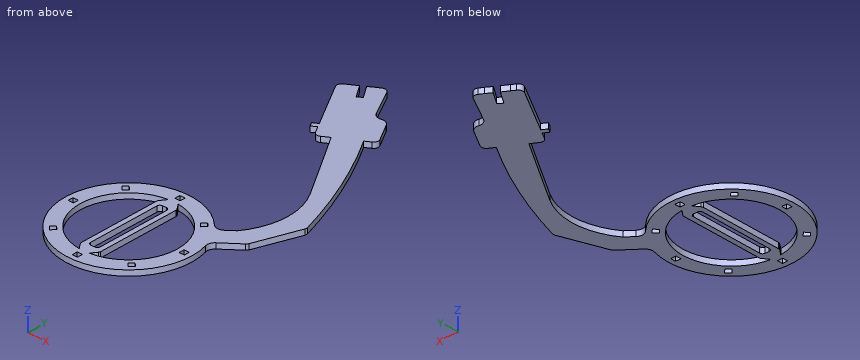
Autodesk Inventor part; units mm, degrees
ref_plane "YZ Plane" through (0, 0, 0) normal (1, 0, 0) x (0, 1, 0)
ref_plane "XZ Plane" through (0, 0, 0) normal (0, 1, 0) x (-1, 0, 0)
ref_plane "XY Plane" through (0, 0, 0) normal (0, 0, 1) x (1, 0, 0)
sketch "Sketch1" plane through (0, 0, 0) normal (0, 0, 1) x (1, 0, 0)
  circle A0 centre (0, 0) radius 65
  dimension "d0" = 130
extrude "Extrusion1" add sketch "Sketch1" along normal blind 5.5
sketch "Sketch5" plane through (0, 0, 5.5) normal (0, 0, 1) x (1, 0, 0)
  line L0 (54.5, 2.75) -> (60, 2.75)
  line L1 (60, 2.75) -> (60, -2.75)
  line L2 (60, -2.75) -> (54.5, -2.75)
  line L3 (54.5, -2.75) -> (54.5, 2.75)
  line L4 (36.5928, 40.4819) -> (40.4819, 44.371)
  line L5 (40.4819, 44.371) -> (44.371, 40.4819)
  line L6 (44.371, 40.4819) -> (40.4819, 36.5928)
  line L7 (40.4819, 36.5928) -> (36.5928, 40.4819)
  line L8 (-2.75, 54.5) -> (-2.75, 60)
  line L9 (-2.75, 60) -> (2.75, 60)
  line L10 (2.75, 60) -> (2.75, 54.5)
  line L11 (2.75, 54.5) -> (-2.75, 54.5)
  line L12 (-40.4819, 36.5928) -> (-44.371, 40.4819)
  line L13 (-44.371, 40.4819) -> (-40.4819, 44.371)
  line L14 (-40.4819, 44.371) -> (-36.5928, 40.4819)
  line L15 (-36.5928, 40.4819) -> (-40.4819, 36.5928)
  line L16 (-54.5, -2.75) -> (-60, -2.75)
  line L17 (-60, -2.75) -> (-60, 2.75)
  line L18 (-60, 2.75) -> (-54.5, 2.75)
  line L19 (-54.5, 2.75) -> (-54.5, -2.75)
  line L20 (-36.5928, -40.4819) -> (-40.4819, -44.371)
  line L21 (-40.4819, -44.371) -> (-44.371, -40.4819)
  line L22 (-44.371, -40.4819) -> (-40.4819, -36.5928)
  line L23 (-40.4819, -36.5928) -> (-36.5928, -40.4819)
  line L24 (2.75, -54.5) -> (2.75, -60)
  line L25 (2.75, -60) -> (-2.75, -60)
  line L26 (-2.75, -60) -> (-2.75, -54.5)
  line L27 (-2.75, -54.5) -> (2.75, -54.5)
  line L28 (40.4819, -36.5928) -> (44.371, -40.4819)
  line L29 (44.371, -40.4819) -> (40.4819, -44.371)
  line L30 (40.4819, -44.371) -> (36.5928, -40.4819)
  line L31 (36.5928, -40.4819) -> (40.4819, -36.5928)
  point P0 (0, 0)
  dimension "d30" = 5.5
  dimension "d31" = 5.5
  dimension "d34" = 360
extrude "Extrusion5" cut sketch "Sketch5" against normal blind 10
sketch "Sketch7" plane through (0, 0, 5.5) normal (0, 0, 1) x (1, 0, 0)
  circle A0 centre (0, 0) radius 65
  line L0 (51.1247, 40.1406) -> (64.8175, 50.8915)
  line L1 (60.6454, 23.3909) -> (84.0046, 41.7313)
  line L2 (84.0046, 41.7313) -> (101.175, 89.1614)
  arc A1 (68.2492, 128.5806) -> (22.61, 201.3724) centre (-8338.3582, -5091.5201) ccw
  arc A2 (101.175, 89.1614) -> (44.4638, 214.134) centre (-401.1925, -63.4539) ccw
  arc A3 (64.8175, 50.8915) -> (68.2492, 128.5806) centre (9.7334, 92.245) ccw
  line L3 (-9.0847, 275.4971) -> (0.0597, 261.7096)
  line L4 (0.0597, 261.7096) -> (-4.5238, 258.6697)
  line L5 (-4.5238, 258.6697) -> (-13.846, 272.7251)
  line L6 (-20.4878, 268.8466) -> (-13.846, 272.7251)
  line L7 (-9.0847, 275.4971) -> (-3.3614, 279.1755)
  line L8 (-20.4878, 268.8466) -> (-29.1232, 263.8039)
  line L9 (-3.3614, 279.1755) -> (5.4134, 283.9717)
  line L10 (11.2184, 194.7202) -> (22.61, 201.3724)
  line L11 (44.4638, 214.134) -> (54.3957, 219.9338)
  line L12 (4.4881, 206.2457) -> (-0.6932, 203.2201)
  line L13 (-0.6932, 203.2201) -> (-3.2145, 207.5378)
  line L14 (-3.2145, 207.5378) -> (1.9667, 210.5634)
  line L15 (-29.1232, 263.8039) -> (1.9667, 210.5634)
  line L16 (4.4881, 206.2457) -> (11.2184, 194.7202)
  line L17 (54.3957, 219.9338) -> (37.2403, 249.3118)
  line L18 (37.2403, 249.3118) -> (27.3211, 243.8901)
  line L19 (27.3211, 243.8901) -> (5.4134, 283.9717)
  dimension "d40" = 250
  dimension "d41" = 20
  dimension "d50" = 5.5
  dimension "d53" = 10
  dimension "d54" = 80
  dimension "d55" = 50
  dimension "d56" = 10
  dimension "d57" = 6
  dimension "d58" = 5
extrude "Extrusion6" add sketch "Sketch7" against normal blind 5.5 contours A0 L0 A3 A1 L10 L16 L12 L13 L14 L15 L8 L6 L5 L4 L3 L7 L9 L19 L18 L17 L11 A2 L2 L1
sketch "Sketch8" plane through (0, 0, 5.5) normal (0, 0, 1) x (1, 0, 0)
  circle A0 centre (0, 0) radius 50
  line L0 (10, 43) -> (10, -43)
  line L1 (-10, -43) -> (-10, 43)
  line L2 (5, 40) -> (-5, 40)
  line L3 (-5, 40) -> (-5, -40)
  line L4 (-5, -40) -> (5, -40)
  line L5 (5, -40) -> (5, 40)
  line L6 (10, -43) -> (5, -49.7494)
  line L7 (-10, -43) -> (-5, -49.7494)
  line L8 (-10, 43) -> (-5, 49.7494)
  line L9 (5, 49.7494) -> (10, 43)
  dimension "d44" = 100
  dimension "d45" = 10
  dimension "d46" = 80
extrude "Extrusion7" cut sketch "Sketch8" against normal blind 5.5 contours A0 L6 L0 L9 | L8 L1 L7 A0 | L5 L4 L3 L2
fillet "Fillet1" radius 3 8 edges at (10, 43, 2.75) (10, -43, 2.75) (-5, 40, 2.75) (-10, -43, 2.75) (5, 40, 2.75) (-10, 43, 2.75) (-5, -40, 2.75) (5, -40, 2.75)
fillet "Fillet2" radius 5 2 edges at (101.175, 89.1614, 2.75) (84.0046, 41.7313, 2.75)
fillet "Fillet3" radius 8 2 edges at (60.6454, 23.3909, 2.75) (51.1247, 40.1406, 2.75)
fillet "Fillet4" radius 5 4 edges at (54.3957, 219.9338, 2.75) (11.2184, 194.7202, 2.75) (5.4134, 283.9717, 2.75) (-29.1232, 263.8039, 2.75)
fillet "Fillet5" radius 8 2 edges at (27.3211, 243.8901, 2.75) (37.2403, 249.3118, 2.75)
properties part number "base"
Verification items for the finished model (mm, model axes). Coordinates: 2 decimals unless noted, no trailing zeros. Loops run counter-clockwise (first coordinate to the right, second up) from the corner with the lowest first, then second, coordinate; pieces in that order, holes last. Notation, with made-up numbers: (14.5, 30.5) -> (53.5, 30.5) arc R10 ccw to (53.5, 42.5) -> close; hole circle Ø3 at (21, 62.25). An arc over 180 degrees is marked (long way). Write each question's results on one line, items separated by ' | '.
Item 1: Section check A-A, the plane y = -20. Enter the section's corners in (x, z), plus the area to 3 significant figures.
Found:
outline: (-61.85, 0) -> (-45.83, 0) -> (-45.83, 5.5) -> (-61.85, 5.5) -> close; (-10, 0) -> (-5, 0) -> (-5, 5.5) -> (-10, 5.5) -> close; (5, 0) -> (10, 0) -> (10, 5.5) -> (5, 5.5) -> close; (45.83, 0) -> (61.85, 0) -> (61.85, 5.5) -> (45.83, 5.5) -> close | area: 231 mm2
Item 2: Material ranges on L1, parallel to X at y = 57, z = 3.5; L2, parallel to Y at x = 23.5, z = 1.25; L3, parallel to Y at x = -42.5, z = 4.05, recorded low to high.
Found:
L1: x = -31.24 to -2.75, 2.75 to 31.24, 68.91 to 89.53 | L2: y = -60.6 to -44.13, 44.13 to 60.6, 199.97 to 250.88 | L3: y = -49.18 to -42.35, -38.61 to -26.34, 26.34 to 38.61, 42.35 to 49.18
Item 3: Section check C-C, the plane y = 143. Enter the section's corners in (x, z), plus the area to 4 significant figures.
Found:
outline: (59.28, 0) -> (81.55, 0) -> (81.55, 5.5) -> (59.28, 5.5) -> close | area: 122.5 mm2
Item 4: Section check D-D, the plane y = 238.5. Enter the section's corners in (x, z), plus the area to 3 significant figures.
Found:
outline: (-14.35, 0) -> (43.55, 0) -> (43.55, 5.5) -> (-14.35, 5.5) -> close | area: 318 mm2
Item 5: Section check B-B, the plane z = 3.45. Count the separate pieces of the cut face and the enclosed holes in it, plus the area to 3 significant figures.
Found:
separate pieces: 1 | enclosed holes: 11 | area: 13,900 mm2
Item 6: Gauge pin test, flat ends, axial feed: pin 1 (2 mm diameter, centred on x = 0.5, z = 3.5, fed in from +Y); pin 2 (1.6 mm diameter, centred on y = 0, z = 3.5, fed in from +X); pin 3 (3 mm diameter, centred on y = 71.5, z = 2.5, fed in from -X); pin 4 (5 mm diameter, centred on x = -11, y = -12.5, fed in from +Z). Record the tip position at first contact, or that the pin passes through.
Found:
pin 1: stops at y = 281.8 | pin 2: stops at x = 65 | pin 3: stops at x = 74.92 | pin 4: stops at z = 5.5
